Read the model definition and answer for the solid it produces. Units are mm, in the model's axes. Face numbers are marked on the shaded views. A direction names the side the tool comes from. Give positions to 0.01 mm unless a question says otherwise; leave off trailing zeros. Write each loop counter-clockwise with the first axis right and the second up, starting at its lowest first coordinate (ties: lowest second). Pieces come first, ordered by that corner, then holes. Notation, with made-up numbers: (60, 13) -> (105, 13) arc R12 ccw to (105, 20) -> close; hole circle Ø9 at (-20, -15.75). An arc over 180 degrees is marked (long way). Use a Markdown table: item, result.
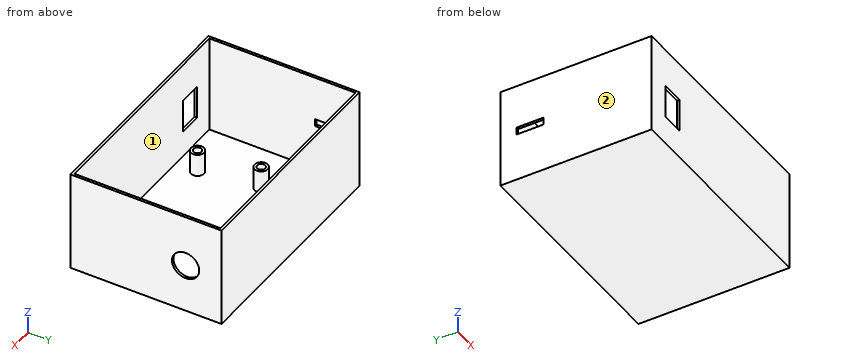
from build123d import *

# Parameters (mm, degrees)
F0_W      = 90
F0_H      = 60
F0_R      = 2.6
F0_R_2    = 1.6
F1_DEPTH  = 40
F2_W      = 88
F2_H      = 58
F3_DEPTH  = 39
F4_DEPTH  = 10
F5_W      = 9.1457683593
F5_H      = 13.2199376822
F6_DEPTH  = 2
F7_W      = 10.7257449999
F7_H      = 2.9699578881
F8_DEPTH  = 2
F9_R      = 5.4148812487
F10_DEPTH = 2


with BuildPart() as f1:
    # F0 (on Top) → F1 (new body)
    with BuildSketch(Plane.XY):
        with Locations((7.6679475605, -1.568697635)):
            Rectangle(F0_W, F0_H)
        with Locations((-14.3958524395, -21.942097635)):
            Circle(F0_R, mode=Mode.SUBTRACT)
        with Locations((33.6609475605, -28.647697635)):
            Circle(F0_R, mode=Mode.SUBTRACT)
        with Locations((-17.7740524395, 1.273502365)):
            Circle(F0_R, mode=Mode.SUBTRACT)
        with Locations((36.3279475605, 12.881302365)):
            Circle(F0_R, mode=Mode.SUBTRACT)
        with Locations((-17.7740524395, 1.273502365)):
            Circle(F0_R)
        with Locations((-17.7740524395, 1.273502365)):
            Circle(F0_R_2, mode=Mode.SUBTRACT)
        with Locations((-14.3958524395, -21.942097635)):
            Circle(F0_R)
        with Locations((-14.3958524395, -21.942097635)):
            Circle(F0_R_2, mode=Mode.SUBTRACT)
        with Locations((33.6609475605, -28.647697635)):
            Circle(F0_R)
        with Locations((33.6609475605, -28.647697635)):
            Circle(F0_R_2, mode=Mode.SUBTRACT)
        with Locations((36.3279475605, 12.881302365)):
            Circle(F0_R)
        with Locations((36.3279475605, 12.881302365)):
            Circle(F0_R_2, mode=Mode.SUBTRACT)
        with Locations((-17.7740524395, 1.273502365)):
            Circle(F0_R_2)
        with Locations((-14.3958524395, -21.942097635)):
            Circle(F0_R_2)
        with Locations((33.6609475605, -28.647697635)):
            Circle(F0_R_2)
        with Locations((36.3279475605, 12.881302365)):
            Circle(F0_R_2)
    extrude(amount=F1_DEPTH)

    # F2 (on face) → F3 (cut)
    with BuildSketch(Plane.XY.offset(40)):
        with Locations((7.6679475605, -1.568697635)):
            Rectangle(F2_W, F2_H)
    extrude(amount=-F3_DEPTH, mode=Mode.SUBTRACT)

    # F0 (on Top) → F4 (join)
    with BuildSketch(Plane.XY):
        with Locations((-14.3958524395, -21.942097635)):
            Circle(F0_R)
        with Locations((-14.3958524395, -21.942097635)):
            Circle(F0_R_2, mode=Mode.SUBTRACT)
        with Locations((-17.7740524395, 1.273502365)):
            Circle(F0_R)
        with Locations((-17.7740524395, 1.273502365)):
            Circle(F0_R_2, mode=Mode.SUBTRACT)
        with Locations((33.6609475605, -28.647697635)):
            Circle(F0_R)
        with Locations((33.6609475605, -28.647697635)):
            Circle(F0_R_2, mode=Mode.SUBTRACT)
        with Locations((36.3279475605, 12.881302365)):
            Circle(F0_R)
        with Locations((36.3279475605, 12.881302365)):
            Circle(F0_R_2, mode=Mode.SUBTRACT)
    extrude(amount=F4_DEPTH)

    # F5 (on face) → F6 (cut)
    with BuildSketch(Plane.XZ.offset(31.568697635)):
        with Locations((-23.679333739, 18.0436503142)):
            Rectangle(F5_W, F5_H)
    extrude(amount=-F6_DEPTH, mode=Mode.SUBTRACT)

    # F7 (on face) → F8 (cut)
    with BuildSketch(Plane(origin=(-37.3320524395, 0, 0), x_dir=(0, -1, 0), z_dir=(-1, 0, 0))):
        with Locations((-16.7629956268, 20.779600367)):
            Rectangle(F7_W, F7_H)
    extrude(amount=-F8_DEPTH, mode=Mode.SUBTRACT)

    # F9 (on face) → F10 (cut)
    with BuildSketch(Plane.YZ.offset(52.6679475605)):
        with Locations((14.1623625532, 19.3200558424)):
            Circle(F9_R)
    extrude(amount=-F10_DEPTH, mode=Mode.SUBTRACT)


solid = f1.part
Item 1: A cutting plane is placed at A-A (y = 20.5). Give the vertices of the cut face in (x, z), then the cut area to 3 significant figures.
Return value:
| item | result |
|---|---|
| outline | (-37.33, 0) -> (52.67, 0) -> (52.67, 40) -> (51.67, 40) -> (51.67, 1) -> (-36.33, 1) -> (-36.33, 19.29) -> (-37.33, 19.29) -> close; (-37.33, 22.26) -> (-36.33, 22.26) -> (-36.33, 40) -> (-37.33, 40) -> close |
| area | 165 mm^2 |
Item 2: A cutting plane is placed at B-B (z = 34). Give the vertices of the cut face in (x, y), then the cut area to 3 significant figures.
Return value:
| item | result |
|---|---|
| outline | (-37.33, -31.57) -> (52.67, -31.57) -> (52.67, 28.43) -> (-37.33, 28.43) -> close; hole (-36.33, -30.57) -> (51.67, -30.57) -> (51.67, 27.43) -> (-36.33, 27.43) -> close |
| area | 296 mm^2 |
Item 3: Straight lines are drawn through the part: line 1 along Y through (x, z) = (6, 37); line 2 along X through (y, z) = (-7, 7); line 3 along Z through (x, y) = (-21, 24.5). For each, find the intervals that lie inside material, in ascending order. Write a range as [from, to].
Return value:
| item | result |
|---|---|
| line 1 | [-31.57, -30.57], [27.43, 28.43] |
| line 2 | [-37.33, -36.33], [51.67, 52.67] |
| line 3 | [0, 1] |
Item 4: A cutting plane is placed at D-D (y = -9). Give the vertices of the cut face in (x, z).
Return value:
| item | result |
|---|---|
| outline | (-37.33, 0) -> (52.67, 0) -> (52.67, 40) -> (51.67, 40) -> (51.67, 1) -> (-36.33, 1) -> (-36.33, 40) -> (-37.33, 40) -> close |
Item 5: A tool of negligible diameter and unlimited length cuts with its end or side. For the marked faces 1 and 2, from which of +Z, -Z, +X, -X, +Y, -Y can it reach the whole face along a straight path? Write none if from no direction.
Return value:
| item | result |
|---|---|
| face 1 | +Z |
| face 2 | +Z, -Z, -X, +Y, -Y |
Item 6: A cutting plane is placed at C-C (x = 26.5). Give the vertices of the cut face in (y, z).
Return value:
| item | result |
|---|---|
| outline | (-31.57, 0) -> (28.43, 0) -> (28.43, 40) -> (27.43, 40) -> (27.43, 1) -> (-30.57, 1) -> (-30.57, 40) -> (-31.57, 40) -> close |
Item 7: Each of these flat-tipped pins is pushed along its axis until it touches: P1, Ø2, axis at x = 17, y = -13, coming from the +Z side; P2, Ø4, axis at x = -18.5, y = 1.5, coming from the +Z side. Where does it stop, or does it pass through?
Return value:
| item | result |
|---|---|
| P1 | z = 1 |
| P2 | z = 10 |
